from build123d import *

# Parameters (mm, degrees)
BOSS_EXTRU_1_DEPTH      = 10
CONG_1_RADIUS           = 5
CONG_1_LENGTH           = 5
CONG_2_RADIUS           = 5
CONG_2_LENGTH           = 5
CONG_3_R                = 10
CONG_4_R                = 10
CONG_6_R                = 3
CONG_7_R                = 3
ESQUISSE2_R             = 1.5
ENL_V_MAT_EXTRU_1_DEPTH = 10
BOSS_EXTRU_2_START      = 21
ESQUISSE3_W             = 5
ESQUISSE3_H             = 2.5
BOSS_EXTRU_2_DEPTH      = 5
ESQUISSE5_R             = 2.5
BOSS_EXTRU_3_DEPTH      = 5
CONG_8_R                = 3
CONG_9_R                = 3
CONG_14_R               = 0.5


with BuildPart() as part:
    # Esquisse1 → Boss.-Extru.1 (new body)
    with BuildSketch(Plane.XY):
        Polygon((0, 0), (16, 0), (16, 20), (31, 20), (31, 0), (47, 0), (47, 5), (36, 5), (36, 25), (11, 25), (11, 5), (0, 5), align=None)
    extrude(amount=BOSS_EXTRU_1_DEPTH)

    # Congé1: full round fillet: the end face becomes a half cylinder, R = half its width
    cong_1_face = Plane((0, 2.5, 5), x_dir=(0, -1, 0), z_dir=(-1, 0, 0))  # on the end face: x along it, z out of the body
    cong_1_slab = cong_1_face.offset(-CONG_1_RADIUS / 2) * Box(CONG_1_LENGTH, 2 * CONG_1_RADIUS, CONG_1_RADIUS, mode=Mode.PRIVATE)  # the body's end, R deep
    cong_1_round = Plane((5, 2.5, 5), x_dir=(-1, 0, 0), z_dir=(0, -1, 0)) * Cylinder(CONG_1_RADIUS, CONG_1_LENGTH, mode=Mode.PRIVATE)  # its axis R under the face
    add(cong_1_slab - cong_1_round, mode=Mode.SUBTRACT)

    # Congé2: full round fillet: the end face becomes a half cylinder, R = half its width
    cong_2_face = Plane((47, 2.5, 5), x_dir=(0, 1, 0), z_dir=(1, 0, 0))  # on the end face: x along it, z out of the body
    cong_2_slab = cong_2_face.offset(-CONG_2_RADIUS / 2) * Box(CONG_2_LENGTH, 2 * CONG_2_RADIUS, CONG_2_RADIUS, mode=Mode.PRIVATE)  # the body's end, R deep
    cong_2_round = Plane((42, 2.5, 5), x_dir=(1, 0, 0), z_dir=(0, 1, 0)) * Cylinder(CONG_2_RADIUS, CONG_2_LENGTH, mode=Mode.PRIVATE)  # its axis R under the face
    add(cong_2_slab - cong_2_round, mode=Mode.SUBTRACT)

    # Congé3
    cong_3_edges = [part.edges().sort_by_distance(p)[0] for p in [
        (31, 0, 5),
        (16, 0, 5),
    ]]
    fillet(cong_3_edges, radius=CONG_3_R)

    # Congé4
    cong_4_edges = [part.edges().sort_by_distance(p)[0] for p in [
        (11, 25, 5),
        (36, 25, 5),
    ]]
    fillet(cong_4_edges, radius=CONG_4_R)

    # Congé6
    cong_6_edges = [part.edges().sort_by_distance(p)[0] for p in [
        (11, 5, 5),
    ]]
    fillet(cong_6_edges, radius=CONG_6_R)

    # Congé7
    cong_7_edges = [part.edges().sort_by_distance(p)[0] for p in [
        (36, 5, 5),
    ]]
    fillet(cong_7_edges, radius=CONG_7_R)

    # Esquisse2 → Enlèv. mat.-Extru.1 (cut)
    with BuildSketch(Plane(origin=(0, 5, 0), x_dir=(1, 0, 0), z_dir=(0, 1, 0))):
        with Locations(Location((5, -5, 0), (0, 0, 270))):
            Circle(ESQUISSE2_R)
        with Locations(Location((42, -5, 0), (0, 0, 270))):
            Circle(ESQUISSE2_R)
    extrude(amount=-ENL_V_MAT_EXTRU_1_DEPTH, mode=Mode.SUBTRACT)

    # Esquisse3 → Boss.-Extru.2 (add)
    with BuildSketch(Plane(origin=(0, 0, 0), x_dir=(0, 0, -1), z_dir=(1, 0, 0)).offset(BOSS_EXTRU_2_START)):
        with Locations((-5, 26.25)):
            Rectangle(ESQUISSE3_W, ESQUISSE3_H)
    extrude(amount=BOSS_EXTRU_2_DEPTH)

    # Esquisse5 → Boss.-Extru.3 (add)
    with BuildSketch(Plane(origin=(26, 0, 0), x_dir=(0, 0, -1), z_dir=(1, 0, 0))):
        with BuildLine():
            Line((-7.5, 27.5), (-2.5, 27.5))
            ThreePointArc((-2.5, 27.5), (-5, 34.622498999), (-7.5, 27.5))
        make_face()
        with Locations((-5, 30.622498999)):
            Circle(ESQUISSE5_R, mode=Mode.SUBTRACT)
    extrude(amount=-BOSS_EXTRU_3_DEPTH)

    # Congé8
    cong_8_edges = [part.edges().sort_by_distance(p)[0] for p in [
        (23.5, 27.5, 7.5),
    ]]
    fillet(cong_8_edges, radius=CONG_8_R)

    # Congé9
    cong_9_edges = [part.edges().sort_by_distance(p)[0] for p in [
        (23.5, 27.5, 2.5),
    ]]
    fillet(cong_9_edges, radius=CONG_9_R)

    # Congé14
    cong_14_edges = [part.edges().sort_by_distance(p)[0] for p in [
        (21, 25.64618599, 2.5),
        (26, 25.64618599, 2.5),
        (21, 25.64618599, 7.5),
        (26, 25.64618599, 7.5),
        (26, 27.274352486, 7.665266452),
        (21, 27.274352486, 7.665266452),
        (21, 34.622498999, 5),
        (26, 34.622498999, 5),
        (21, 27.274352486, 2.334733548),
        (26, 27.274352486, 2.334733548),
    ]]
    fillet(cong_14_edges, radius=CONG_14_R)


solid = part.part
The listing builds one solid part. Answer for the finished solid, in the listing's coordinates (mm). A direction names the side the tool comes from. Round coordinates to 2 decimals unless told otherwise and drop trailing zeros. Write each loop counter-clockwise with the first axis right and the second up, starting at its lowest first coordinate (ties: lowest second). Pieces come first, ordered by that corner, then holes. Notation, with made-up numbers: (-4, -20) - (32, -20) arc R26 cw to (32, 10) - close; hole circle Ø1 at (79, 45). An arc over 180 degrees is marked (long way). Use a Markdown table: item, result. Add a question column.
1. The part is cut by section C-C (y = 17.5). Write down the section's boundary in (x, z).
2. For a pull along Y with two mould halves and no side action, classify faces 1 (the face through (33.85, 3.01, 5.07)), 2 (the face through (23.53, 27.29, 7.67)), 3 (the face through (24, 25, 1)), 4 (the face through (10.14, 5.9, 5.07)) as +Y half, -Y half, draft (parallel to the pull), parting line (faces both ways), or undercut.
3. The part is cut by section B-B (z = 5). Give the number of separate pieces and of enclosed holes in the cut face, and give its area (3 significant figures).
4. Consider line 1 (X direction, y = 3.55, z = 5); line 2 (X direction, y = 4.5, z = 5.25); line 3 (Y direction, x = 44, z = 7.25). Determine where each line is inside the solid, lowest interval first.
5. Flat-ended cylindrical pins translate along their axes: P1, Ø2.5, axis at x = 44, z = 4, coming from the +Y side; P2, Ø5, axis at y = 21.5, z = 5.5, coming from the -X side; P3, Ø0.9, axis at x = 24, z = 1, coming from the +Y side. Find the tip coordinate at first contact, or state that the pin passes through.
6. A tool of negligible diameter and unlimited length cuts with its end or side. For faces 5 (the face through (21, 27.6, 5)), 6 (the face through (12.99, 2.85, 5.07)), 7 (the face through (36, 11, 5)), from which of +Z, -Z, +X, -X, +Y, -Y can it reach the whole face along a straight path? Write none if from no direction.
7. The part is cut by section D-D (x = 34). Write down the section's boundary in (y, z), and give its area (3 significant figures).
8. The part is cut by section A-A (y = 5.5). Write down the section's boundary in (x, z).
Reported:
| question | item | result |
|---|---|---|
| 1 | outline | (11.32, 0) - (16, 0) - (16, 10) - (11.32, 10) - close; (31, 0) - (35.68, 0) - (35.68, 10) - (31, 10) - close |
| 2 | face 1 | -Y half |
| 2 | face 2 | undercut |
| 2 | face 3 | undercut |
| 2 | face 4 | +Y half |
| 3 | separate pieces | 4 |
| 3 | enclosed holes | 0 |
| 3 | area | 346 mm^2 |
| 4 | line 1 | 0 to 3.5, 6.5 to 13.64, 33.36 to 40.5, 43.5 to 47 |
| 4 | line 2 | 0.01 to 3.52, 6.48 to 14.35, 32.65 to 40.52, 43.48 to 46.99 |
| 4 | line 3 | 0 to 5 |
| 5 | P1 | y = 5 |
| 5 | P2 | x = 11.83 |
| 5 | P3 | y = 32.47 |
| 6 | face 5 | +Z, -Z, -X, +Y |
| 6 | face 6 | +Z, -Z, -Y |
| 6 | face 7 | +Z, -Z, +X, +Y |
| 7 | outline | (2.86, 0) - (21, 0) - (21, 10) - (2.86, 10) - close |
| 7 | area | 181 mm^2 |
| 8 | outline | (9.66, 0) - (14.93, 0) - (14.93, 10) - (9.66, 10) - close; (32.07, 0) - (37.34, 0) - (37.34, 10) - (32.07, 10) - close |
